from build123d import *

# Parameters (mm, degrees)
SKETCH1_W            = 16
SKETCH1_H            = 8
BOSS_EXTRUDE1_DEPTH  = 9.6
SHELL1_T             = -1.6
BOSS_EXTRUDE3_DEPTH  = 16
SKETCH2_R            = 2.4
BOSS_EXTRUDE2_DEPTH  = 1.6
LPATTERN1_COUNT      = 2
LPATTERN1_PITCH      = 8
LPATTERN1_COUNT_DIR2 = 3
LPATTERN1_PITCH_DIR2 = 8


with BuildPart() as part:
    # Sketch1 → Boss-Extrude1 (new body)
    with BuildSketch(Plane(origin=(0, 0, 0), x_dir=(1, 0, 0), z_dir=(0, 1, 0))):
        with Locations((8, 4)):
            Rectangle(SKETCH1_W, SKETCH1_H)
    extrude(amount=BOSS_EXTRUDE1_DEPTH)

    # Shell1
    shell1_openings = [part.faces().sort_by_distance(p)[0] for p in [
        (8, 0, -4),
    ]]
    offset(amount=SHELL1_T, openings=shell1_openings, kind=Kind.INTERSECTION)

    # Sketch3 → Boss-Extrude3 (add)
    with BuildSketch(Plane(origin=(16, 0, 0), x_dir=(0, 0, -1), z_dir=(1, 0, 0))):
        Polygon((8, 0), (24, 9.6), (8, 9.6), align=None)
    extrude(amount=-BOSS_EXTRUDE3_DEPTH)

    # Sketch2 → Boss-Extrude2 (add)
    with BuildSketch(Plane(origin=(0, 9.6, 0), x_dir=(1, 0, 0), z_dir=(0, 1, 0))):
        with Locations(Location((12, 4, 0), (0, 0, 90))):
            Circle(SKETCH2_R)
    boss_extrude2 = extrude(amount=BOSS_EXTRUDE2_DEPTH)

    # LPattern1: Boss-Extrude2 2 × 3
    with Locations(*[(-i * LPATTERN1_PITCH, 0, -j * LPATTERN1_PITCH_DIR2) for i in range(LPATTERN1_COUNT) for j in range(LPATTERN1_COUNT_DIR2) if (i, j) != (0, 0)]):
        add(boss_extrude2)


solid = part.part
Design review of the part built by this model. Coordinates are the model's own, in mm. A direction names the side the tool comes from. Coordinates: 2 decimals unless noted, no trailing zeros. Loops run counter-clockwise (first coordinate to the right, second up) from the corner with the lowest first, then second, coordinate; pieces in that order, holes last. Notation, with made-up numbers: (-12, 81.5) -> (12, 81.5) arc R25 ccw to (12, 111.5) -> close; hole circle Ø7 at (-4.75, 51.25). An arc over 180 degrees is marked (long way). Use a Markdown table: item, result. Add a question column.
Item 1: The part is to be moulded in two halves that separate along X. For faces 4 (the flat face through (16, 6, -9)), 5 (the flat face through (1.6, 4, -4)), 6 (the flat face through (12, 11.2, -12)), say which applies: +X half, -X half, draft (parallel to the pull), parting line (faces both ways), or undercut.
Item 2: Wall thickness on L1, parallel to Z at x = 5, y = 10.5; L2, parallel to Z at x = 8.75, y = 1.5; L3, parallel to Y at x = 9, z = -4.5: over which ranges is each line inside the solid? List them lowest first. Write a range as from..to.
Item 3: We need section C-C, the plane x = 12. Write out the cut boundary in (y, z), and give its area (3 significant figures).
Item 4: We need section D-D, the plane z = -20. Write out the cut boundary in (x, y), and give its area (3 significant figures).
Item 5: We need section A-A, the plane y = 3. Write out the cut boundary in (x, z), and give its area (3 significant figures).
Item 6: Clearance check with flat-ended pins moving along their axes: P1, Ø6.5, axis at x = 11, y = 2.5, coming from the -Z side; P2, Ø6, axis at x = 2, z = -11.5, coming from the -Y side; P3, Ø1, axis at x = 13, y = 8.5, coming from the -Z side. State where each tip first meets the part, or that it passes through.
Item 7: Machinability: for faces 1 (the cylindrical face through (9.976, 10.389, -5.29)), 2 (the flat face through (12, 11.2, -20)), 3 (the flat face through (14.4, 4, -4)), which of the approach directions +Z, -Z, +X, -X, +Y, -Y give a long, thin tool a straight path to every point of the face, cutting with its end or side? Answer none if there is none.
Item 8: We need section B-B, the plane z = -12. Write out the cut boundary in (x, y), and give its area (3 significant figures).
Numbers:
| question | item | result |
|---|---|---|
| 1 | face 4 | +X half |
| 1 | face 5 | undercut |
| 1 | face 6 | draft |
| 2 | L1 | z = -22.18..-17.82, -14.18..-9.82, -6.18..-1.82 |
| 2 | L2 | z = -10.5..-6.4, -1.6..0 |
| 2 | L3 | y = 8..9.6 |
| 3 | outline | (0, -8) -> (9.6, -24) -> (9.6, -22.4) -> (11.2, -22.4) -> (11.2, -17.6) -> (9.6, -17.6) -> (9.6, -14.4) -> (11.2, -14.4) -> (11.2, -9.6) -> (9.6, -9.6) -> (9.6, -6.4) -> (11.2, -6.4) -> (11.2, -1.6) -> (9.6, -1.6) -> (9.6, 0) -> (0, 0) -> (0, -1.6) -> (8, -1.6) -> (8, -6.4) -> (0, -6.4) -> close |
| 3 | area | 138 mm^2 |
| 4 | outline | (0, 7.2) -> (16, 7.2) -> (16, 9.6) -> (14.4, 9.6) -> (14.4, 11.2) -> (9.6, 11.2) -> (9.6, 9.6) -> (6.4, 9.6) -> (6.4, 11.2) -> (1.6, 11.2) -> (1.6, 9.6) -> (0, 9.6) -> close |
| 4 | area | 53.8 mm^2 |
| 5 | outline | (0, -13) -> (16, -13) -> (16, 0) -> (0, 0) -> close; hole (1.6, -6.4) -> (14.4, -6.4) -> (14.4, -1.6) -> (1.6, -1.6) -> close |
| 5 | area | 147 mm^2 |
| 6 | P1 | stops at z = -17.58 |
| 6 | P2 | stops at y = 0.3 |
| 6 | P3 | stops at z = -23 |
| 7 | face 1 | +Y |
| 7 | face 2 | +Z, -Z, +X, -X, +Y |
| 7 | face 3 | -Y |
| 8 | outline | (0, 2.4) -> (16, 2.4) -> (16, 9.6) -> (14.4, 9.6) -> (14.4, 11.2) -> (9.6, 11.2) -> (9.6, 9.6) -> (6.4, 9.6) -> (6.4, 11.2) -> (1.6, 11.2) -> (1.6, 9.6) -> (0, 9.6) -> close |
| 8 | area | 131 mm^2 |
